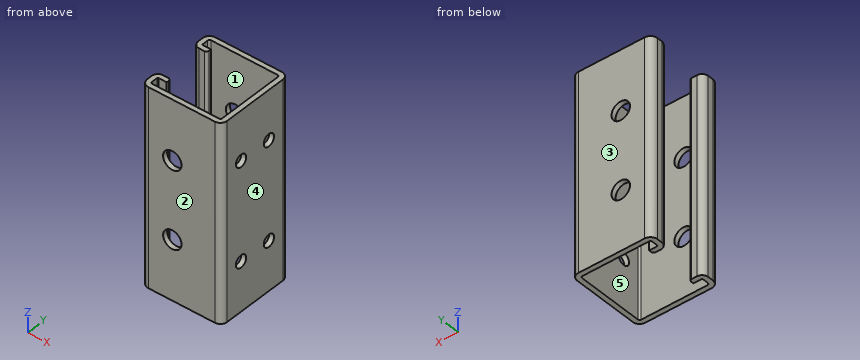
from build123d import *

# Parameters (mm, degrees)
BOSS_EXTRUDE1_DEPTH      = 50.8
BOSS_EXTRUDE1_DEPTH_BACK = 50.8
SKETCH7_R                = 4.7625
CUT_EXTRUDE1_DEPTH       = 45.72
SKETCH8_R                = 3.175
CUT_EXTRUDE2_DEPTH       = 2.54


with BuildPart() as part:
    # Sketch4 → Boss-Extrude1 (new, two sides: drawn at the far end of the back side and taken through both)
    with BuildSketch(Plane.XY.offset(-BOSS_EXTRUDE1_DEPTH_BACK)):
        with BuildLine():
            Line((-17.0815, -20.6375), (17.17675, -20.6375))
            ThreePointArc((17.17675, -20.6375), (19.623869793, -19.623869793), (20.6375, -17.17675))
            Line((20.6375, -17.17675), (20.6375, 17.17675))
            ThreePointArc((20.6375, 17.17675), (19.623869793, 19.623869793), (17.17675, 20.6375))
            Line((17.17675, 20.6375), (-17.0815, 20.6375))
            ThreePointArc((-17.0815, 20.6375), (-19.595971714, 19.595971714), (-20.6375, 17.0815))
            Line((-20.6375, 17.0815), (-20.6375, 14.2875))
            ThreePointArc((-20.6375, 14.2875), (-19.70756403, 12.04243597), (-17.4625, 11.1125))
            Line((-17.4625, 11.1125), (-14.7701, 11.1125))
            ThreePointArc((-14.7701, 11.1125), (-13.872074388, 11.484474388), (-13.5001, 12.3825))
            Line((-13.5001, 12.3825), (-13.5001, 13.6525))
            Line((-13.5001, 13.6525), (-17.5895, 13.6525))
            ThreePointArc((-17.5895, 13.6525), (-17.948710245, 13.801289755), (-18.0975, 14.1605))
            Line((-18.0975, 14.1605), (-18.0975, 17.0815))
            ThreePointArc((-18.0975, 17.0815), (-17.79992049, 17.79992049), (-17.0815, 18.0975))
            Line((-17.0815, 18.0975), (17.17675, 18.0975))
            ThreePointArc((17.17675, 18.0975), (17.827818569, 17.827818569), (18.0975, 17.17675))
            Line((18.0975, 17.17675), (18.0975, -17.17675))
            ThreePointArc((18.0975, -17.17675), (17.827818569, -17.827818569), (17.17675, -18.0975))
            Line((17.17675, -18.0975), (-17.0815, -18.0975))
            ThreePointArc((-17.0815, -18.0975), (-17.79992049, -17.79992049), (-18.0975, -17.0815))
            Line((-18.0975, -17.0815), (-18.0975, -14.1605))
            ThreePointArc((-18.0975, -14.1605), (-17.948710245, -13.801289755), (-17.5895, -13.6525))
            Line((-17.5895, -13.6525), (-13.5001, -13.6525))
            Line((-13.5001, -13.6525), (-13.5001, -12.3825))
            ThreePointArc((-13.5001, -12.3825), (-13.872074388, -11.484474388), (-14.7701, -11.1125))
            Line((-14.7701, -11.1125), (-17.4625, -11.1125))
            ThreePointArc((-17.4625, -11.1125), (-19.70756403, -12.04243597), (-20.6375, -14.2875))
            Line((-20.6375, -14.2875), (-20.6375, -17.0815))
            ThreePointArc((-20.6375, -17.0815), (-19.595971714, -19.595971714), (-17.0815, -20.6375))
        make_face()
    extrude(amount=BOSS_EXTRUDE1_DEPTH + BOSS_EXTRUDE1_DEPTH_BACK)

    # Sketch7 → Cut-Extrude1 (cut)
    with BuildSketch(Plane(origin=(0, 20.6375, 0), x_dir=(1, 0, 0), z_dir=(0, 1, 0))):
        with Locations(Location((-4.73075, -20, 0), (0, 0, 180))):
            Circle(SKETCH7_R)
        with Locations(Location((-4.73075, 20, 0), (0, 0, 180))):
            Circle(SKETCH7_R)
    extrude(amount=-CUT_EXTRUDE1_DEPTH, mode=Mode.SUBTRACT)

    # Sketch8 → Cut-Extrude2 (cut)
    with BuildSketch(Plane(origin=(20.6375, 0, 0), x_dir=(0, 0, -1), z_dir=(1, 0, 0))):
        with Locations(Location((25.4, -8.588375, 0), (0, 0, 90))):
            Circle(SKETCH8_R)
        with Locations(Location((25.4, 8.588375, 0), (0, 0, 180))):
            Circle(SKETCH8_R)
        with Locations(Location((-25.4, -8.588375, 0), (0, 0, 180))):
            Circle(SKETCH8_R)
        with Locations(Location((-25.4, 8.588375, 0), (0, 0, 90))):
            Circle(SKETCH8_R)
    extrude(amount=-CUT_EXTRUDE2_DEPTH, mode=Mode.SUBTRACT)


solid = part.part
Model file for the job. Use its own axes, mm. Face numbers are marked on the shaded views. A direction names the side the tool comes from. Give positions to 0.01 mm unless a question says otherwise; leave off trailing zeros. Order: outer loops, then holes, each group sorted by start corner. A loop starts at its lowest first (then second) coordinate and runs counter-clockwise, first axis right, second up. Notation, with made-up numbers: (66.5, -12) - (96.5, -12) arc R12 cw to (96.5, -4) - close; hole circle Ø1 at (86.25, 39). An arc over 180 degrees is marked (long way). Write item = value, one per line. Start each with the question number.
1. Probe line 1 along Y through (x, z) = (-16.5, 32.5); line 2 along Y through (x, z) = (3, 36.5). List the from-to ranges inside material, lowest first.
2. Cut at C-C, the plane x = -6. List the corners of the cut face in (y, z).
3. Which spindle directions (+Z, -Z, +X, -X, +Y, -Y) get a long thin tool onto all of the face, cutting with end or side? Do the marked faces 1 and 2. Say none if no direction does.
4. Two-plate mould, pull along Y, no slides. Class the marked faces 3, 4 and 5: pulls with the +Y half, pulls with the -Y half, needs draft (parallel to the pull), parting line crosses it, or undercut.
5. Cut at D-D, the plane y = -0.5. List the corners of the cut face in (x, z), and give its area (3 significant figures).
6. Drop flat-ended pins along their axis: P1, Ø15, axis at x = -4.73, z = -20, coming from the +Y side; P2, Ø8.5, axis at x = -4.73, z = -20, coming from the +Y side; P3, Ø7.5, axis at y = -8.59, z = 25.4, coming from the -X side; P4, Ø3, axis at y = 12.5, z = 0.5, coming from the -X side. Give the stop position or say it passes through.
7. Cut at A-A, the plane x = 15.5. List the corners of the cut face in (y, z), and give its area (3 significant figures).
Taken from the geometry:
q1.line_1 = -20.64 to -18.1, -13.65 to -11.11, 11.11 to 13.65, 18.1 to 20.64
q1.line_2 = -20.64 to -18.1, 18.1 to 20.64
q2.outline = (-20.64, -50.8) - (-18.1, -50.8) - (-18.1, -24.59) - (-20.64, -24.59) - close; (-20.64, -15.41) - (-18.1, -15.41) - (-18.1, 15.41) - (-20.64, 15.41) - close; (-20.64, 24.59) - (-18.1, 24.59) - (-18.1, 50.8) - (-20.64, 50.8) - close; (18.1, -50.8) - (20.64, -50.8) - (20.64, -24.59) - (18.1, -24.59) - close; (18.1, -15.41) - (20.64, -15.41) - (20.64, 15.41) - (18.1, 15.41) - close; (18.1, 24.59) - (20.64, 24.59) - (20.64, 50.8) - (18.1, 50.8) - close
q3.face_1 = +Z, -Z
q3.face_2 = +Z, -Z, +X, -X, -Y
q4.face_3 = pulls with the +Y half
q4.face_4 = needs draft
q4.face_5 = undercut
q5.outline = (18.1, -50.8) - (20.64, -50.8) - (20.64, 50.8) - (18.1, 50.8) - close
q5.area = 258 mm²
q6.P1 = 20.64
q6.P2 = through
q6.P3 = -19.97
q6.P4 = -20.62
q7.outline = (-20.64, -50.8) - (-18.1, -50.8) - (-18.1, 50.8) - (-20.64, 50.8) - close; (18.1, -50.8) - (20.64, -50.8) - (20.64, 50.8) - (18.1, 50.8) - close
q7.area = 516 mm²
